Autodesk Inventor part; units mm, degrees
ref_plane "body_to_dummy_XY" through (0, 0, 0) normal (0, -1, 0) x (1, 0, 0)
ref_plane "body_to_dummy_YZ" through (0, 0, 0) normal (1, 0, 0) x (0, 0, 1)
ref_plane "body_to_dummy_ZX" through (0, 0, 0) normal (0, 0, 1) x (0, -1, 0)
sketch "Sketch_1" plane through (0, 0, 0) normal (1, 0, 0) x (0, 1, 0)
  line L0 (-56, 0) -> (0, 0)
  line L1 (-3.2, 0) -> (-3.2, -28.075)
  line L2 (-3.2, -28.075) -> (-5.8, -25.22)
  line L3 (-5.8, -25.22) -> (-5.8, -25.7879)
  line L4 (-5.8, -25.7879) -> (-7.8, -25.7879)
  line L5 (-7.8, -25.7879) -> (-7.8, -24.1)
  arc A0 (-10.6, -25.5) -> (-7.8, -24.1) centre (-10.6, -22) ccw
  line L6 (-10.6, -25.5) -> (-29.936, -25.5)
  arc A1 (-51.0993, -18.3) -> (-29.936, -25.5) centre (-29.936, 9.203) ccw
  line L7 (-51.0993, -18.3) -> (-56, -18.3)
  line L8 (-56, -18.3) -> (-56, 0)
  line L9 (-56, 0) -> (-3.2, 0)
revolve "Revolution1" add sketch "Sketch_1" angle 360 about axis through (0, -56, 0) along (0, -1, 0)
sketch "Sketch_2" plane through (0, 0, 0) normal (0, 0, 1) x (1, 0, 0)
  line L0 (-50, -13.191) -> (-21.7584, -56)
  line L1 (-21.7584, -56) -> (-17.7584, -56)
  line L2 (-17.7584, -56) -> (-17.7584, -13.191)
  line L3 (-17.7584, -13.191) -> (-50, -13.191)
extrude "Extrusion1" cut sketch "Sketch_2" along normal mid plane 56
sketch "Sketch_3" plane through (0, 0, 0) normal (0, 0, 1) x (1, 0, 0)
  line L0 (-150, -150) -> (150, -150)
  line L1 (150, -150) -> (150, 150)
  line L2 (150, 150) -> (-150, 150)
  line L3 (-150, 150) -> (-150, -150)
  arc A0 (-37.3451, -41.2613) -> (-18.215, -51.6199) centre (-27, -45) ccw
  line L4 (-18.215, -51.6199) -> (3.8878, -22.2883)
  arc A1 (13.4715, -17.51) -> (3.8878, -22.2883) centre (13.4715, -29.51) ccw
  line L5 (13.4715, -17.51) -> (27.5, -17.51)
  line L6 (27.5, -17.51) -> (27.5, 0)
  line L7 (27.5, 0) -> (-28.7615, 0)
  line L8 (-28.7615, 0) -> (-28.7615, -17.51)
  line L9 (-28.7615, -17.51) -> (-37.3451, -41.2613)
sketch "Sketch_5" plane through (-17.7584, 0, 0) normal (1, 0, 0) x (0, 0, -1)
  line L0 (-18.3, -56) -> (-16.3, -56)
  line L1 (-16.3, -56) -> (-16.3, -17.501)
  line L2 (-16.3, -17.501) -> (16.3, -17.501)
  line L3 (16.3, -17.501) -> (16.3, -56)
  line L4 (16.3, -56) -> (18.3, -56)
  line L5 (18.3, -56) -> (18.3, -13.191)
  line L6 (18.3, -13.191) -> (-18.3, -13.191)
  line L7 (-18.3, -13.191) -> (-18.3, -56)
extrude "Extrusion2" add sketch "Sketch_5" along normal mid plane 44
extrude "Extrusion3" cut sketch "Sketch_3" along normal mid plane 100
sketch "Sketch_4" plane through (0, -5.8, 0) normal (0, 1, 0) x (1, 0, 0)
  circle A0 centre (0, 0) radius 24
extrude "Extrusion4" cut sketch "Sketch_4" against normal blind 24.076
sketch "Sketch_6" plane through (0, 0, 0) normal (1, 0, 0) x (0, 1, 0)
  line L0 (-56, 0) -> (0, 0)
  line L1 (-29.6366, 0) -> (-29.6366, -24)
  line L2 (-29.6366, -24) -> (-29.936, -24)
  arc A0 (-51.0993, -16.8) -> (-29.936, -24) centre (-29.936, 10.703) ccw
  line L3 (-51.0993, -16.8) -> (-51.0993, 0)
  line L4 (-51.0993, 0) -> (-29.6366, 0)
revolve "Revolution2" cut sketch "Sketch_6" angle 360 about axis through (0, -56, 0) along (0, -1, 0)
sketch "Sketch_7" plane through (0, 0, 0) normal (1, 0, 0) x (0, 1, 0)
  line L0 (-56, 16.3) -> (-56, -16.3)
  line L1 (-56, -16.3) -> (-17.501, -16.3)
  line L2 (-17.501, -16.3) -> (-17.501, 16.3)
  line L3 (-17.501, 16.3) -> (-56, 16.3)
extrude "Extrusion5" cut sketch "Sketch_7" along normal mid plane 116
sketch "Sketch_8" plane through (0, 0, 0) normal (0, 0, 1) x (1, 0, 0)
  line L0 (-50, -15.3345) -> (-25.5, -13.191)
  line L1 (-25.5, -13.191) -> (-50, -13.191)
  line L2 (-50, -13.191) -> (-50, -15.3345)
extrude "Extrusion6" cut sketch "Sketch_8" along normal mid plane 116
sketch "Sketch_9" plane through (0, 0, 0) normal (0, 0, 1) x (1, 0, 0)
  circle A0 centre (-27, -45) radius 4
extrude "Extrusion7" add sketch "Sketch_9" along normal mid plane 36.6
sketch "Sketch_10" plane through (-27, 0, 0) normal (1, 0, 0) x (0, 0, -1)
  line L0 (19.8, -45) -> (18.3, -45)
  line L1 (18.3, -45) -> (18.3, -39)
  arc A0 (19.8, -40.5) -> (18.3, -39) centre (18.3, -40.5) ccw
  line L2 (19.8, -40.5) -> (19.8, -45)
  line L3 (19.8, -45) -> (18.3, -45)
revolve "Revolution3" add sketch "Sketch_10" angle 360 about axis through (-27, -45, -19.8) along (0, 0, -1)
ref_plane "body_to_dummy_XY" through (0, 0, 0) normal (0, -1, 0) x (1, 0, 0)
ref_plane "body_to_dummy_YZ" through (0, 0, 0) normal (1, 0, 0) x (0, 0, 1)
ref_plane "body_to_dummy_ZX" through (0, 0, 0) normal (0, 0, 1) x (0, -1, 0)
ref_plane "body_to_stopper_left_XY" through (-27, -45, -18.3) normal (0, 0, -1) x (1, 0, 0)
ref_plane "body_to_stopper_left_YZ" through (-27, -45, -18.3) normal (1, 0, 0) x (0, -1, 0)
ref_plane "body_to_stopper_left_ZX" through (-27, -45, -18.3) normal (0, -1, 0) x (0, 0, -1)
ref_plane "body_to_stopper_right_XY" through (-27, -45, 18.3) normal (0, 0, 1) x (1, 0, 0)
ref_plane "body_to_stopper_right_YZ" through (-27, -45, 18.3) normal (1, 0, 0) x (0, 1, 0)
ref_plane "body_to_stopper_right_ZX" through (-27, -45, 18.3) normal (0, 1, 0) x (0, 0, 1)
ref_plane "body_to_swivel_XY" through (0, -3.2, 0) normal (0, -1, 0) x (1, 0, 0)
ref_plane "body_to_swivel_YZ" through (0, -3.2, 0) normal (1, 0, 0) x (0, 0, 1)
ref_plane "body_to_swivel_ZX" through (0, -3.2, 0) normal (0, 0, 1) x (0, -1, 0)
ref_plane "body_to_wheel_XY" through (-27, -45, 0) normal (0, 0, 1) x (1, 0, 0)
ref_plane "body_to_wheel_YZ" through (-27, -45, 0) normal (1, 0, 0) x (0, 1, 0)
ref_plane "body_to_wheel_ZX" through (-27, -45, 0) normal (0, 1, 0) x (0, 0, 1)
properties part number "BODY-HSMCS50"
Design review of the part built by this model. Coordinates are the model's own, in mm. A direction names the side the tool comes from. Round coordinates to 2 decimals unless told otherwise and drop trailing zeros. Order: outer loops, then holes, each group sorted by start corner. A loop starts at its lowest first (then second) coordinate and runs counter-clockwise, first axis right, second up.
1) Clearance check with flat-ended pins moving along their axes: pin 1 Ø4.5 at (y, z) = (-15.5, -7.5) entering from -X; pin 2 Ø12.5 at (x, y) = (-25, -39) entering from -Z; pin 3 Ø4 at (x, z) = (13, 4) entering from -Y. State where each tip first meets the part, or that it passes through.
The answers:
pin 1: stops at x = -28.76
pin 2: stops at z = -19.8
pin 3: stops at y = -5.8
2) Consider section B-B (x = 0). State the section outline as (y, z) points (3 decimals).
The answers:
outline: (-27.448, -25.5) - (-10.6, -25.5) arc R3.5 ccw to (-7.8, -24.1) - (-7.8, -25.788) - (-5.8, -25.788) - (-5.8, -25.22) - (-3.2, -28.075) - (-3.2, 28.075) - (-5.8, 25.22) - (-5.8, 25.788) - (-7.8, 25.788) - (-7.8, 24.1) arc R3.5 ccw to (-10.6, 25.5) - (-27.448, 25.5) - (-27.448, 24) - (-5.8, 24) - (-5.8, -24) - (-27.448, -24) - close
3) Machinability: for faces 1 (the cylindrical face through (-27.521, -41.034, 0.228)), 2 (the flat face through (16, -17.51, -19)), 3 (the flat face through (-28.762, -15, 0)), which of the approach directions +Z, -Z, +X, -X, +Y, -Y give a long, thin tool a straight path to every point of the face, cutting with its end or side? Answer none if there is none.
The answers:
face 1: none
face 2: +Z, -Z, +X, -Y
face 3: +Z, -Z, -X, +Y
4) Draft analysis for pull direction Z (two halves, no side actions). For faces 4 (the flat face through (16, -17.51, 19)), 5 (the cylindrical face through (7.746, -6.814, -24.597)), 6 (the flat face through (-26, -37, -16.3)), state which applies: released by +Z, released by -Z, zero draft, split by the parting line, or undercut.
The answers:
face 4: zero draft
face 5: split by the parting line
face 6: undercut
5) For L1, parallel to Z at x = 0, y = -17.25; L2, parallel to X at y = -10, z = 0; L3, parallel to Z at x = -33.5, y = -50, list the stretches that pass through material, from the lowest coordinate up.
The answers:
L1: z = -25.5 to -24, 24 to 25.5
L2: x = -25.45 to -24, 24 to 25.45
L3: z = -18.3 to -16.3, 16.3 to 18.3
6) Consider section A-A (y = -25). State the section outline as (x, z) points.
The answers:
outline: (-31.47, -18.3) - (-17.76, -18.3) arc R25.5 ccw to (1.84, -25.43) - (1.84, -23.93) arc R24 cw to (-17.62, -16.3) - (-31.47, -16.3) - close; (-31.47, 16.3) - (-17.62, 16.3) arc R24 cw to (1.84, 23.93) - (1.84, 25.43) arc R25.5 ccw to (-17.76, 18.3) - (-31.47, 18.3) - close
